Geometry check sheet. Reference: the model listing, model coordinates, mm. Face numbers are marked on the shaded views. A direction names the side the tool comes from. Coordinates: 2 decimals unless noted, no trailing zeros. Write each loop counter-clockwise with the first axis right and the second up, starting at its lowest first coordinate (ties: lowest second). Pieces come first, ordered by that corner, then holes. Notation, with made-up numbers: (8.5, -7.75) -> (30.5, -7.75) arc R23 ccw to (30.5, 3.25) -> close; hole circle Ø8 at (5, 72.5). An arc over 180 degrees is marked (long way). Answer as CSV lines item,"result".
```python
from build123d import *


with BuildPart() as f1:
    # F0 (on Front) → F1 (revolve)
    with BuildSketch(Plane.XZ):
        with BuildLine():
            Line((0, -9), (10, -9))
            Line((10, -9), (10, -7))
            Line((10, -7), (12, -7))
            Line((12, -7), (12, -6))
            Line((12, -6), (10, -4))
            Line((10, -4), (10, -2))
            Line((10, -2), (12, -2))
            Line((12, -2), (12, -1))
            Line((12, -1), (10, 1))
            Line((10, 1), (10, 3))
            Line((10, 3), (12, 3))
            Line((12, 3), (12, 4))
            Line((12, 4), (10, 6))
            Line((10, 6), (10, 11))
            Line((10, 11), (14, 11))
            Line((14, 11), (14, 12))
            ThreePointArc((14, 12), (7.561179, 16.232774), (0, 17.717143))
            Line((0, 17.717143), (0, -9))
        make_face()
    revolve(axis=Axis((0, 0, 4.358572), (0, 0, -1)))


solid = f1.part
```
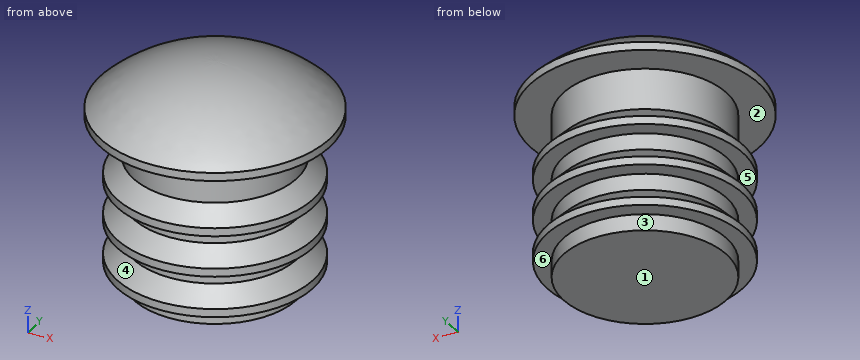
Item 1: Set-up check for the marked faces 1 and 2: record each of +Z, -Z, +X, -X, +Y, -Y from which the full face is reachable in a straight line by a thin tool's end or side.
Responses:
face 1,"-Z, +X, -X, +Y, -Y"
face 2,"none"
Item 2: Release check for a two-part mould opening along Z. For the marked faces 3, 4, 5 and 6 record: +Z half, -Z half, draft (parallel to the pull), parting line (faces both ways), or undercut.
Responses:
face 3,"draft"
face 4,"undercut"
face 5,"undercut"
face 6,"-Z half"
Item 3: Thickness scan on probe 1 along Z at (x, y) = (-9, 6); probe 2 along Z at (x, y) = (-9.25, 6); probe 3 along X at (y, z) = (-2.75, -5.5). Record the ranges inside material, lowest first.
Responses:
probe 1,"z = -7 to -4.82, -2 to 0.18, 3 to 5.18, 11 to 14.54"
probe 2,"z = -7 to -5.03, -2 to -0.03, 3 to 4.97, 11 to 14.4"
probe 3,"x = -11.17 to 11.17"
Item 4: Cross-section at A-A, the plane z = 9.25. Record the cut outline in (x, y).
Responses:
outline,"circle Ø20 at (0, 0)"
Item 5: Depth check by flat-ended pin: pin 1 Ø6 at (y, z) = (-9, 5) entering from -X; pin 2 Ø1.5 at (x, y) = (2.5, 3.5) entering from +Z; pin 3 Ø12 at (y, z) = (0, 1) entering from +X. Enter the tip coordinate at first touch or a pass-through.
Responses:
pin 1,"stops at x = -10.29"
pin 2,"stops at z = 17.4"
pin 3,"stops at x = 12"
